Build history of the part. All positions in model axes, mm. A direction names the side the tool comes from. Round coordinates to 2 decimals unless told otherwise and drop trailing zeros. Write each loop counter-clockwise with the first axis right and the second up, starting at its lowest first coordinate (ties: lowest second). Pieces come first, ordered by that corner, then holes. Notation, with made-up numbers: (5, -10) -> (12, -10) arc R6 ccw to (12, 1) -> close; hole circle Ø2 at (50, 17). An arc over 180 degrees is marked (long way). Return JSON: item names as keys, results as strings.
from build123d import *

# Parameters (mm, degrees)
SKETCH1_R           = 10.2
BOSS_EXTRUDE1_DEPTH = 0.95
SKETCH2_R           = 7.8
BOSS_EXTRUDE2_DEPTH = 3.55
SKETCH3_R           = 5.2
CUT_EXTRUDE1_DEPTH  = 2.5
SKETCH4_R           = 3.9
CUT_EXTRUDE2_DEPTH  = 16.110592311


with BuildPart() as part:
    # Sketch1 → Boss-Extrude1 (new body)
    with BuildSketch(Plane.XY.offset(0.95)):
        Circle(SKETCH1_R)
    extrude(amount=-BOSS_EXTRUDE1_DEPTH)

    # Sketch2 → Boss-Extrude2 (add)
    with BuildSketch(Plane.XY.offset(0.95)):
        with Locations(Location((0, 0, 0), (0, 0, 180))):
            Circle(SKETCH2_R)
    extrude(amount=BOSS_EXTRUDE2_DEPTH)

    # Sketch3 → Cut-Extrude1 (cut)
    with BuildSketch(Plane.XY.offset(4.5)):
        Circle(SKETCH3_R)
    extrude(amount=-CUT_EXTRUDE1_DEPTH, mode=Mode.SUBTRACT)

    # Sketch4 → Cut-Extrude2 (cut, through all)
    with BuildSketch(Plane(origin=(0, 0, 0), x_dir=(-1, 0, 0), z_dir=(0, 0, -1))):
        Circle(SKETCH4_R)
    extrude(amount=-CUT_EXTRUDE2_DEPTH, mode=Mode.SUBTRACT)


solid = part.part
Q1. 3-axis set-ups, long thin cutter, end or side, ignore diameter. For faces 1 (the cylindrical face through (5.75, -5.27, 2.7)), 2 (the flat face through (-2, 5, 4.5)): which of +Z, -Z, +X, -X, +Y, -Y reach the whole face in a straight line?
Verdict:
{"face 1": "+Z", "face 2": "+Z, +X, -X, +Y, -Y"}
Q2. Pin check, flat tips, straight feed: pin 1 Ø1 at (x, z) = (2, 1) entering from +Y; pin 2 Ø2 at (x, z) = (5.5, 1.5) entering from +Y. Stop position of each tip, or through.
Verdict:
{"pin 1": "stops at y = 10.09", "pin 2": "stops at y = 9.07"}
Q3. Wall check: L1, parallel to X at y = 0.25, z = 3.25; L2, parallel to Y at x = 0, z = 1.2; L3, parallel to X at y = 1, z = 0.25. Give the ranges that are in metal, low to high.
Verdict:
{"L1": "x = -7.8 to -5.19, 5.19 to 7.8", "L2": "y = -7.8 to -3.9, 3.9 to 7.8", "L3": "x = -10.15 to -3.77, 3.77 to 10.15"}
Q4. Two-plate mould, pull along Y, no slides. Class faces 3 (the cylindrical face through (-0.677, 5.156, 3.268)), 4 (the flat face through (-2, -8, 0.95)), 5 (the cylindrical face through (4.707, -9.049, 0.482)): +Y half, -Y half, draft (parallel to the pull), parting line (faces both ways), or undercut.
Verdict:
{"face 3": "undercut", "face 4": "draft", "face 5": "parting line"}
Q5. Saw through at D-D on x = -7.5. List the corners of the cut face in (y, z).
Verdict:
{"outline": "(-6.91, 0) -> (6.91, 0) -> (6.91, 0.95) -> (2.14, 0.95) -> (2.14, 4.5) -> (-2.14, 4.5) -> (-2.14, 0.95) -> (-6.91, 0.95) -> close"}
Q6. Saw through at B-B on x = 1.25. List the corners of the cut face in (y, z).
Verdict:
{"outline": "(-10.12, 0) -> (-3.69, 0) -> (-3.69, 2) -> (-5.05, 2) -> (-5.05, 4.5) -> (-7.7, 4.5) -> (-7.7, 0.95) -> (-10.12, 0.95) -> close; (3.69, 0) -> (10.12, 0) -> (10.12, 0.95) -> (7.7, 0.95) -> (7.7, 4.5) -> (5.05, 4.5) -> (5.05, 2) -> (3.69, 2) -> close"}
Q7. Saw through at C-C on z = 1.5. List the corners of the cut face in (x, y), then the cut area to 3 significant figures.
Verdict:
{"outline": "circle Ø15.6 at (0, 0); hole circle Ø7.8 at (0, 0)", "area": "143 mm²"}
Q8. Saw through at A-A on y = -2.25. List the corners of the cut face in (x, z), then the cut area to 3 significant figures.
Verdict:
{"outline": "(-9.95, 0) -> (-3.19, 0) -> (-3.19, 2) -> (-4.69, 2) -> (-4.69, 4.5) -> (-7.47, 4.5) -> (-7.47, 0.95) -> (-9.95, 0.95) -> close; (3.19, 0) -> (9.95, 0) -> (9.95, 0.95) -> (7.47, 0.95) -> (7.47, 4.5) -> (4.69, 4.5) -> (4.69, 2) -> (3.19, 2) -> close", "area": "35.7 mm²"}
